Can you work these out from the model? Positions are in its coordinate system, mm. A direction names the side the tool comes from. Round coordinates to 2 decimals unless told otherwise and drop trailing zeros. Write each loop counter-clockwise with the first axis right and the second up, starting at its lowest first coordinate (ties: lowest second). Pieces come first, ordered by that corner, then holes.
Q1. I'm going to push a flat-ended pin straight in: pin 1 Ø1.8 at (x, y) = (-30, 0) entering from +Z. Where does the tip first touch, or does it pass through?
Q2. If we section it at A-A (y = 0): Please give me the cut outline in (x, z), plus the area to 3 significant figures.
Q3. For faces 1 (the flat face through (-30, 0, -22)), 2 (the cylindrical face through (-29, 0, 30)), 3 (the flat face through (-1, 0, 37)), which set-ups out of +Z, -Z, +X, -X, +Y, -Y let a thin tool reach every point of the face, with its end or its side?
Q4. Please list where these lines run through material, in increasing order: line 1 along Y through (x, z) = (30, -25); line 2 along Z through (x, y) = (30.5, -0.75).
Q5. If we section it at B-B (x = 30): Please give me the cut outline in (y, z), plus the area to 3 significant figures.
Q6. We'd pull the mould along Y, two halves only. Please class faces 4 (the flat face through (1, 5, -1)), 5 (the flat face through (30, 0, 22)), 6 (the flat face through (-1, 0, -37)): +Y half, -Y half, draft (parallel to the pull), parting line (faces both ways), or undercut.
Solid Edge part; units mm, degrees
sketch "Sketch1" plane through (0, 0, 0) normal (0, 0, 1) x (1, 0, 0)
  line L0 (-40, -5) -> (40, -5)
  line L1 (40, -5) -> (40, 5)
  line L2 (40, 5) -> (-40, 5)
  line L3 (-40, 5) -> (-40, -5)
  dimension "D1" = 40
  dimension "D2" = 40
extrude "Protrusion1" add sketch "Sketch1" along normal mid plane 74
sketch "Sketch2" plane through (0, 0, 37) normal (0, 0, 1) x (1, 0, 0)
  circle A0 centre (-30, 0) radius 1
  circle A1 centre (30, 0) radius 1
  dimension "D1" = 30
extrude "Extrusionsausschnitt_1" cut sketch "Sketch2" against normal blind 15
mirror "Mirror1" about plane through (0, 0, 0) normal (0, 0, 1) of "Extrusionsausschnitt_1"
properties material "Nylon, allgemein"
A:
1. pin 1: stops at z = 22
2. outline: (-40, -37) - (-31, -37) - (-31, -22) - (-29, -22) - (-29, -37) - (29, -37) - (29, -22) - (31, -22) - (31, -37) - (40, -37) - (40, 37) - (31, 37) - (31, 22) - (29, 22) - (29, 37) - (-29, 37) - (-29, 22) - (-31, 22) - (-31, 37) - (-40, 37) - close
2. area: 5,800 mm2
3. face 1: -Z
3. face 2: +Z
3. face 3: +Z, +X, -X, +Y, -Y
4. line 1: y = -5 to -1, 1 to 5
4. line 2: z = -22 to 22
5. outline: (-5, -37) - (-1, -37) - (-1, -22) - (1, -22) - (1, -37) - (5, -37) - (5, 37) - (1, 37) - (1, 22) - (-1, 22) - (-1, 37) - (-5, 37) - close
5. area: 680 mm2
6. face 4: +Y half
6. face 5: undercut
6. face 6: draft
